```python
from build123d import *

# Parameters (mm, degrees)
F0_W      = 3
F0_H      = 30
F1_DEPTH  = 70
F2_W      = 1.5
F2_H      = 15
F3_DEPTH  = 70
F5_DEPTH  = 8.8
F6_DEPTH  = 25
F7_DEPTH  = 25
F8_DEPTH  = 13
F9_W      = 0.1
F9_H      = 58.1
F10_DEPTH = 15
F12_DEPTH = 130
F14_DEPTH = 130
F15_R     = 8
F17_W     = 1.6
F17_H     = 18.1
F16_W     = 1.6
F16_H     = 18.1
F18_DEPTH = 1.1
F20_DEPTH = 44.7


with BuildPart() as f1:
    # F0 (on Top) → F1 (new body)
    with BuildSketch(Plane.XY):
        Rectangle(F0_W, F0_H)
    extrude(amount=F1_DEPTH)

    # F2 (on face) → F3 (cut)
    with BuildSketch(Plane.XY.offset(70)):
        with Locations((-0.75, 7.5)):
            Rectangle(F2_W, F2_H)
    extrude(amount=-F3_DEPTH, mode=Mode.SUBTRACT)

    # F4 (on face) → F5 (join)
    with BuildSketch(Plane(origin=(0, 0, 0), x_dir=(-1, 0, 0), z_dir=(0, 1, 0))):
        with BuildLine():
            Line((1.5, 33.833809621), (1.5, 36.166190379))
            ThreePointArc((1.5, 36.166190379), (0.8349366084, 36.7067163971), (0, 36.9))
            Line((0, 36.9), (0, 33.1))
            ThreePointArc((0, 33.1), (0.8349366084, 33.2932836029), (1.5, 33.833809621))
        make_face()
    extrude(amount=F5_DEPTH)

    # F6 (add): a face of the model
    f6_faces = [f1.faces().sort_by_distance(p)[0] for p in [
        (0.25, -2.5, 0),
    ]]
    extrude(f6_faces, amount=F6_DEPTH)

    # F7 (add): a face of the model
    f7_faces = [f1.faces().sort_by_distance(p)[0] for p in [
        (0.25, -2.5, 70),
    ]]
    extrude(f7_faces, amount=F7_DEPTH)

    # F8 (add): a face of the model
    f8_faces = [f1.faces().sort_by_distance(p)[0] for p in [
        (0, -15, 35),
    ]]
    extrude(f8_faces, amount=F8_DEPTH)

    # F9 (on face) → F10 (cut)
    with BuildSketch(Plane(origin=(0, 15, 0), x_dir=(-1, 0, 0), z_dir=(0, 1, 0))):
        with Locations((-0.05, 65.95)):
            Rectangle(F9_W, F9_H)
        with Locations((-0.05, 4.05)):
            Rectangle(F9_W, F9_H)
    extrude(amount=-F10_DEPTH, mode=Mode.SUBTRACT)

    # F11 (on face) → F12 (cut)
    with BuildSketch(Plane(origin=(0, 0, -25), x_dir=(1, 0, 0), z_dir=(0, 0, -1))):
        Polygon((-1.7338935286, -15.3450844809), (0.3, -15), (0.1, -15), (0.1, -14.7996032594), (-1.6308530467, -13.0653167143), align=None)
    extrude(amount=-F12_DEPTH, mode=Mode.SUBTRACT)

    # F13 (on face) → F14 (cut)
    with BuildSketch(Plane(origin=(0, 0, -25), x_dir=(1, 0, 0), z_dir=(0, 0, -1))):
        Polygon((0.1, -14.7832093728), (0.0735654176, -14.7755583748), (-0.2710041881, -15.1656661183), (0.654931704, -15.2749568224), (1.0070909047, -15.0457499549), (0.8490225115, -15), (0.1, -15), align=None)
        Polygon((0.8490225115, -15), (0.1, -14.7832093728), (0.1, -15), align=None)
    extrude(amount=-F14_DEPTH, mode=Mode.SUBTRACT)

    # F15
    f15_edges = [f1.edges().sort_by_distance(p)[0] for p in [
        (0, -28, 95),
        (0, -28, -25),
    ]]
    fillet(f15_edges, radius=F15_R)

    # F17 (on face) + F16 (on face) → F18 (cut)
    with BuildSketch(Plane(origin=(0, 0, 0), x_dir=(-1, 0, 0), z_dir=(0, 1, 0))):
        with Locations((0.7, 4.1168239134)):
            Rectangle(F17_W, F17_H)
    with BuildSketch(Plane(origin=(0, 0, 0), x_dir=(-1, 0, 0), z_dir=(0, 1, 0))):
        with Locations((0.7, 65.8831760866)):
            Rectangle(F16_W, F16_H)
    extrude(amount=-F18_DEPTH, mode=Mode.SUBTRACT)

    # F19 (on Top) → F20 (cut)
    with BuildSketch(Plane.XY):
        Polygon((-4.6543548815, 8.3620538935), (-2.3670103401, 7.1775359102), (0, 8.7909307331), (-4.6543548815, 10.0162932649), align=None)
    extrude(amount=F20_DEPTH, mode=Mode.SUBTRACT)


solid = f1.part
```
Input: part model. Units: mm. Frame: model coordinates. A direction names the side the tool comes from. Round coordinates to 2 decimals unless told otherwise and drop trailing zeros. Order: outer loops, then holes, each group sorted by start corner. A loop starts at its lowest first (then second) coordinate and runs counter-clockwise, first axis right, second up. Notation, with made-up numbers: (-39.75, 64.5) - (10.25, 64.5) arc R23 cw to (10.25, 103.5) - close; hole circle Ø8 at (27.25, -39.75). An arc over 180 degrees is marked (long way). Answer in a Markdown table with one row per item.
Item 1: Pin query (flat end, axial travel): pin 1 (5 mm diameter, centred on y = 5, z = 76.5, fed in from -X); pin 2 (1.3 mm diameter, centred on x = -0.5, z = 68.5, fed in from +Y); pin 3 (1.3 mm diameter, centred on x = -1, z = 84, fed in from +Y). Return the tip coordinate at first contact, or that it passes through.
Model answer:
| item | result |
|---|---|
| pin 1 | stops at x = 0.1 |
| pin 2 | stops at y = 14.8 |
| pin 3 | stops at y = 0 |
Item 2: Section query D-D (z = 40). Return the cut outline in (x, y), then the cut area to 3 significant figures.
Model answer:
| item | result |
|---|---|
| outline | (-1.5, -28) - (1.5, -28) - (1.5, 15) - (0.85, 15) - (0.1, 14.78) - (0.1, 0) - (-1.5, 0) - close |
| area | 105 mm² |
Item 3: Reachability of faces 1 (the flat face through (0, 12, 35)), 2 (the flat face through (0, -6, 95)) from +Z, -Z, +X, -X, +Y, -Y: full face, straight path, thin tool, end or side. Return the list, or none.
Model answer:
| item | result |
|---|---|
| face 1 | +Z, -Z, -X, +Y |
| face 2 | +Z, +X, -X, +Y, -Y |
Item 4: Section query A-A (z = 10). Return the cut outline in (x, y).
Model answer:
| item | result |
|---|---|
| outline | (-1.5, -28) - (1.5, -28) - (1.5, 15) - (0.85, 15) - (0.1, 14.78) - (0.1, -1.1) - (-1.5, -1.1) - close |
Item 5: Section query C-C (x = -0.75). Return the cut outline in (y, z), then the cut area to 3 significant figures.
Model answer:
| item | result |
|---|---|
| outline | (-28, -17) arc R8 ccw to (-20, -25) - (0, -25) - (0, -4.93) - (-1.1, -4.93) - (-1.1, 13.17) - (0, 13.17) - (0, 33.25) - (8.28, 33.25) - (8.28, 36.75) - (0, 36.75) - (0, 56.83) - (-1.1, 56.83) - (-1.1, 74.93) - (0, 74.93) - (0, 95) - (-20, 95) arc R8 ccw to (-28, 87) - close |
| area | 3,320 mm² |
Item 6: Section query B-B (y = 11.5). Return the cut outline in (x, z), then the cut area to 3 significant figures.
Model answer:
| item | result |
|---|---|
| outline | (0, 33.1) - (0.1, 33.1) - (0.1, -25) - (1.5, -25) - (1.5, 95) - (0.1, 95) - (0.1, 36.9) - (0, 36.9) - close |
| area | 168 mm² |
Item 7: Line query: line 1 (Y direction, x = -0.8, z = 54.5); line 2 (X direction, y = 2, z = 80); line 3 (Y direction, x = -0.75, z = 13). Output: solid intervals per line, ascending.
Model answer:
| item | result |
|---|---|
| line 1 | y = -28 to 0 |
| line 2 | x = 0.1 to 1.5 |
| line 3 | y = -28 to -1.1 |
